Geometry check sheet. Reference: the model listing, model coordinates, mm. Face numbers are marked on the shaded views. Round coordinates to 2 decimals unless told otherwise and drop trailing zeros. Loops run counter-clockwise (first coordinate to the right, second up) from the corner with the lowest first, then second, coordinate; pieces in that order, holes last. Notation, with made-up numbers: (-3, 38) - (29, 38) arc R27 cw to (29, 56) - close; hole circle Ø4 at (-40, -25). An arc over 180 degrees is marked (long way). Answer as CSV lines item,"result". Start each with the question number.
1) Cross-section at C-C on y = -57.5. Record the boundary of the cut face in (x, z).
2) Cross-section at B-B on y = -146. Record the boundary of the cut face in (x, z), and give its area (3 significant figures).
3) Cross-section at A-A on x = 0. Record the boundary of the cut face in (y, z), and give its area (3 significant figures).
4) Thickness scan on line 1 along Y through (x, z) = (6, 1); line 2 along Z through (x, y) = (0, -49.5); line 3 along Z through (x, y) = (0, -143.5). Record the ranges inside material, lowest first.
5) Draft check along Y on the marked faces 1, 2 and 3. Enter one of: released by +Y, released by -Y, zero draft, split by the parting line, or undercut.
6) Depth check by flat-ended pin: P1, Ø4, axis at x = -11, y = -130, coming from the +Z side; P2, Ø4, axis at x = 4, z = 8.5, coming from the -Y side; P3, Ø1.5, axis at y = -124, z = 11.5, coming from the +X side. Enter the tip coordinate at first touch or a pass-through.
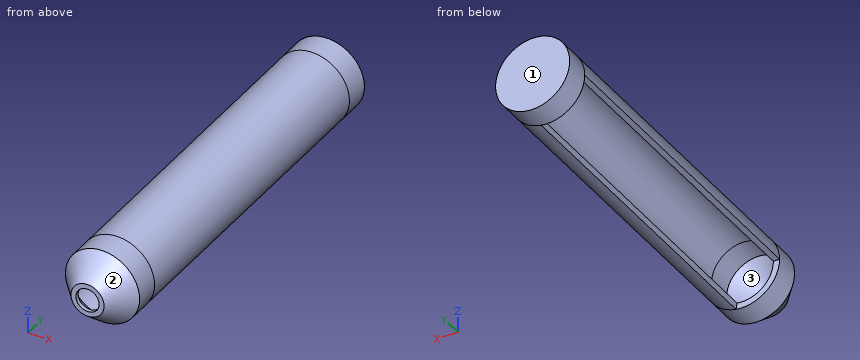
from build123d import *

# Parameters (mm, degrees)
REVOLVE2_ANGLE = 260.00000000000057


with BuildPart() as part:
    # Sketch1 → Revolve1 (revolve)
    with BuildSketch(Plane.XY, mode=Mode.PRIVATE) as revolve1_sk:
        Polygon((-12.499999999999998, -10), (0, -10), (0, 0), (-15, 0), (-14.999999999999998, -10.000000000000002), align=None)
        Polygon((-12.499999999999982, -150), (-12.499999999999984, -140), (-14.999999999999982, -140), (-14.999999999999982, -150), (-6.693376137081884, -159.99999999999997), (-4.693376137081883, -160), (-4.693376137081885, -158.5), (-6.335585997031014, -158.5), align=None)
    revolve(revolve1_sk.sketch.rotate(Axis((3.2365e-12, -943.5188438052121, 0), (-3.43e-15, 1, 0)), 180), axis=Axis((3.2365e-12, -943.5188438052121, 0), (-3.43e-15, 1, 0)))

    # Sketch1_5 → Revolve2 (revolve)
    with BuildSketch(Plane.XY):
        Polygon((-12.499999999999998, -10), (-15, -10.000000000000002), (-14.999999999999984, -140), (-12.499999999999984, -140), align=None)
    revolve(axis=Axis((3.2365e-12, -943.5188438052121, 0), (-3.43e-15, 1, 0)), revolution_arc=REVOLVE2_ANGLE)


solid = part.part
Answer block:
1,outline,"(-15, 0) - (-12.5, 0) arc R12.5 cw (long way) to (2.17, -12.31) - (2.6, -14.77) arc R15 ccw (long way) to start"
2,outline,"circle Ø30 at (0, 0); hole circle Ø25 at (0, 0)"
2,area,"216 mm^2"
3,outline,"(-160, -6.69) - (-150, -15) - (-140, -15) - (-140, -12.5) - (-150, -12.5) - (-158.5, -6.34) - (-158.5, -4.69) - (-160, -4.69) - close; (-160, 4.69) - (-158.5, 4.69) - (-158.5, 6.34) - (-150, 12.5) - (-10, 12.5) - (-10, -15) - (0, -15) - (0, 15) - (-150, 15) - (-160, 6.69) - close"
3,area,"718 mm^2"
4,line 1,"y = -160 to -158.5, -10 to 0"
4,line 2,"z = 12.5 to 15"
4,line 3,"z = -15 to -12.5, 12.5 to 15"
5,face 1,"released by +Y"
5,face 2,"released by -Y"
5,face 3,"undercut"
6,P1,"stops at z = 12"
6,P2,"stops at y = -159.16"
6,P3,"stops at x = 10.46"
